Geometry: see drawing. Coordinates: mm, zero at the bounding-box minimum. Round coordinates to 2 decimals unless told otherwise and drop trailing zeros. Loops run counter-clockwise (first coordinate to the right, second up) from the corner with the lowest first, then second, coordinate; pieces in that order, holes last. Notation, with made-up numbers: (80, 50) -> (93, 50) arc R17 ccw to (93, 77) -> close; hole circle Ø9 at (-30.75, 21). An arc over 180 degrees is marked (long way). Answer in a Markdown table with one row per item.
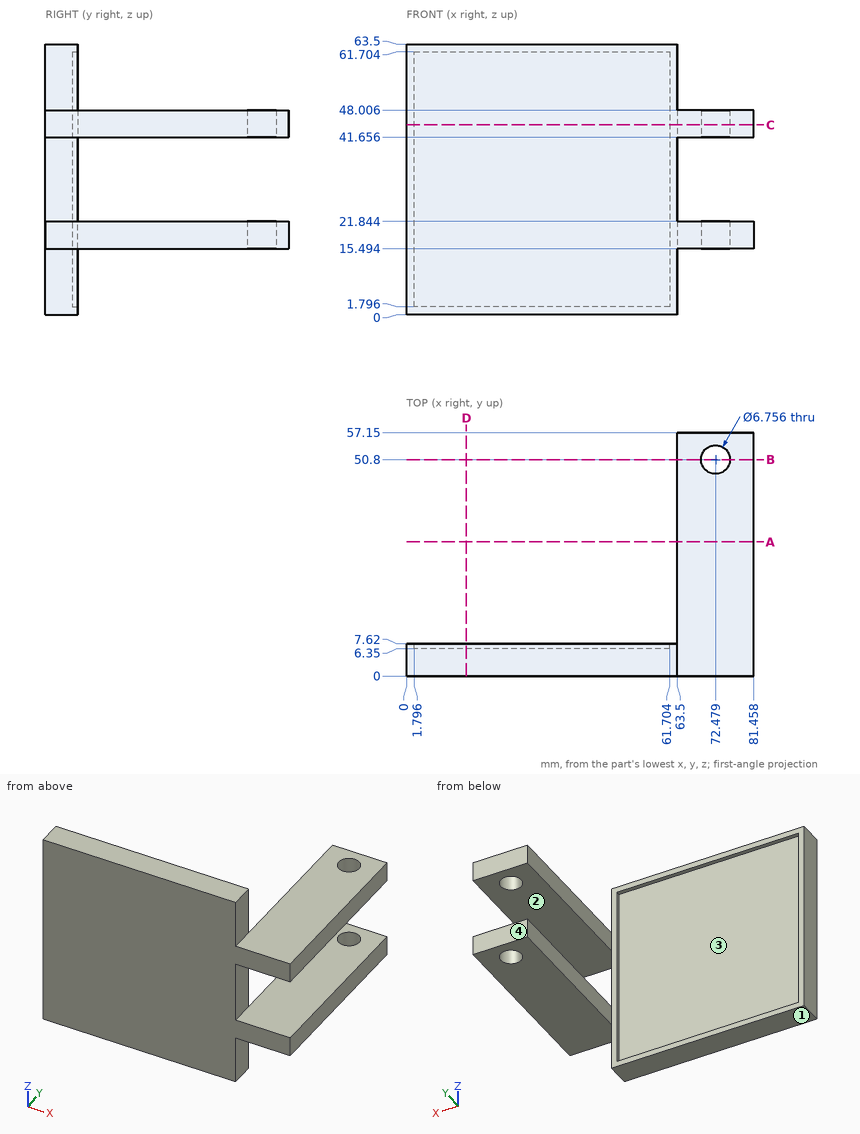
Item 1: Section query B-B, the plane y = 50.8. Output: boundary loops of the cut face in (x, z), and give its area (3 significant figures).
Ans:
| item | result |
|---|---|
| outline | (63.5, 15.49) -> (69.1, 15.49) -> (69.1, 21.84) -> (63.5, 21.84) -> close; (63.5, 41.66) -> (69.1, 41.66) -> (69.1, 48.01) -> (63.5, 48.01) -> close; (75.86, 15.49) -> (81.46, 15.49) -> (81.46, 21.84) -> (75.86, 21.84) -> close; (75.86, 41.66) -> (81.46, 41.66) -> (81.46, 48.01) -> (75.86, 48.01) -> close |
| area | 142 mm2 |
Item 2: Ray query, L1, parallel to X at y = 50.8, z = 17.5; L2, parallel to Z at x = 73, y = 39; L3, parallel to Y at x = 11.5, z = 27.5. Return the intervals inside material, ascending.
Ans:
| item | result |
|---|---|
| L1 | 63.5 to 69.1, 75.86 to 81.46 |
| L2 | 15.49 to 21.84, 41.66 to 48.01 |
| L3 | 0 to 6.35 |
Item 3: First-contact query: P1, Ø1.9, axis at y = 39, z = 43.5, coming from the -X side; P2, Ø1.5, axis at x = 73, y = 40, coming from the -Z side; P3, Ø8.5, axis at y = 4, z = 35, coming from the +X side. Flat tips, straight axial feed; report the tip coordinate or a pass-through.
Ans:
| item | result |
|---|---|
| P1 | x = 63.5 |
| P2 | z = 15.49 |
| P3 | x = 63.5 |
Item 4: Section query A-A, the plane y = 31.5. Output: boundary loops of the cut face in (x, z).
Ans:
| item | result |
|---|---|
| outline | (63.5, 15.49) -> (81.46, 15.49) -> (81.46, 21.84) -> (63.5, 21.84) -> close; (63.5, 41.66) -> (81.46, 41.66) -> (81.46, 48.01) -> (63.5, 48.01) -> close |
Item 5: Section query C-C, the plane z = 44.5. Output: boundary loops of the cut face in (x, y).
Ans:
| item | result |
|---|---|
| outline | (0, 0) -> (81.46, 0) -> (81.46, 57.15) -> (63.5, 57.15) -> (63.5, 7.62) -> (61.7, 7.62) -> (61.7, 6.35) -> (1.8, 6.35) -> (1.8, 7.62) -> (0, 7.62) -> close; hole circle Ø6.76 at (72.48, 50.8) |
Item 6: Mould query, pull axis Z, two halves, no side actions, for the marked faces 1, 2, 3 and 4. Classes: released by +Z, released by -Z, zero draft, split by the parting line, or undercut.
Ans:
| item | result |
|---|---|
| face 1 | released by -Z |
| face 2 | undercut |
| face 3 | undercut |
| face 4 | zero draft |
Item 7: Section query D-D, the plane x = 14. Output: boundary loops of the cut face in (y, z).
Ans:
| item | result |
|---|---|
| outline | (0, 0) -> (7.62, 0) -> (7.62, 1.8) -> (6.35, 1.8) -> (6.35, 61.7) -> (7.62, 61.7) -> (7.62, 63.5) -> (0, 63.5) -> close |
